from build123d import *

# Parameters (mm, degrees)
SKETCH_1_R          = 2
EXTRUDE_1_DEPTH     = 5
SKETCH_2_R          = 2.5
EXTRUDE_2_DEPTH     = 30
SKETCH_3_R          = 3.5
EXTRUDE_3_DEPTH     = 4
CUT_EXTRUDE_1_DEPTH = 3


with BuildPart() as part:
    # Эскиз1 → Бобышка-Вытянуть1 (new body)
    with BuildSketch(Plane.XY):
        Circle(SKETCH_1_R)
    extrude(amount=EXTRUDE_1_DEPTH)

    # Эскиз2 → Бобышка-Вытянуть2 (add)
    with BuildSketch(Plane.XY.offset(5)):
        Circle(SKETCH_2_R)
    extrude(amount=EXTRUDE_2_DEPTH)

    # Эскиз3 → Бобышка-Вытянуть3 (add)
    with BuildSketch(Plane.XY.offset(35)):
        Circle(SKETCH_3_R)
    extrude(amount=EXTRUDE_3_DEPTH)

    # Эскиз4 → Вырез-Вытянуть1 (cut)
    with BuildSketch(Plane.XY.offset(39)):
        Polygon((1.5, 0.866025404), (0, 1.732050808), (-1.5, 0.866025404), (-1.5, -0.866025404), (0, -1.732050808), (1.5, -0.866025404), align=None)
    extrude(amount=-CUT_EXTRUDE_1_DEPTH, mode=Mode.SUBTRACT)


solid = part.part
Check sheet for the modelled part. Datum: model origin and axes. Units: mm. A direction names the side the tool comes from. Give positions to 0.01 mm unless a question says otherwise; leave off trailing zeros. Write each loop counter-clockwise with the first axis right and the second up, starting at its lowest first coordinate (ties: lowest second). Pieces come first, ordered by that corner, then holes. Notation, with made-up numbers: (-2, 67) -> (6, 67) arc R24 cw to (6, 103) -> close; hole circle Ø10 at (-26, 10.5). An arc over 180 degrees is marked (long way). One line per item, written item: value. Start each with the question number.
Item 1: Section check C-C on z = 6. Record the cut outline in (x, y).
Item 2: Section check B-B on x = -0.5. Record the cut outline in (y, z).
Item 3: Section check A-A on y = 0. Record the cut outline in (x, z).
Item 4: Draft check along Y on faces 4 (the cylindrical face through (-0.54, -2.44, 19.79)), 5 (the flat face through (-0.74, 1.305, 37.521)), 6 (the flat face through (2, -2, 35)). Enter one of: +Y half, -Y half, draft (parallel to the pull), parting line (faces both ways), or undercut.
Item 5: Material ranges on probe 1 along X at (y, z) = (2, 31.5); probe 2 along X at (y, z) = (1.5, 10), recorded low to high. Write a range as from..to.
Item 6: Gauge pin test, flat ends, axial feed: pin 1 (0.9 mm diameter, centred on x = 0, y = 0, fed in from +Z); pin 2 (1 mm diameter, centred on y = 0.5, z = 25.5, fed in from -X). Record the tip position at first contact, or that the pin passes through.
Item 7: Section check D-D on y = 3. Record the cut outline in (x, z).
Item 8: Tool access check on faces 1 (the flat face through (-1, 2, 5)), 2 (the cylindrical face through (3.233, -1.341, 36.972)), 3 (the flat face through (0.74, -1.305, 37.521)). Record the directions out of +Z, -Z, +X, -X, +Y, -Y that give a thin tool (end or side, any length) a straight path to the whole face; none if there is none.
Results list:
1. outline: circle Ø5 at (0, 0)
2. outline: (-3.46, 35) -> (-2.45, 35) -> (-2.45, 5) -> (-1.94, 5) -> (-1.94, 0) -> (1.94, 0) -> (1.94, 5) -> (2.45, 5) -> (2.45, 35) -> (3.46, 35) -> (3.46, 39) -> (1.44, 39) -> (1.44, 36) -> (-1.44, 36) -> (-1.44, 39) -> (-3.46, 39) -> close
3. outline: (-3.5, 35) -> (-2.5, 35) -> (-2.5, 5) -> (-2, 5) -> (-2, 0) -> (2, 0) -> (2, 5) -> (2.5, 5) -> (2.5, 35) -> (3.5, 35) -> (3.5, 39) -> (1.5, 39) -> (1.5, 36) -> (-1.5, 36) -> (-1.5, 39) -> (-3.5, 39) -> close
4. face 4: parting line
4. face 5: undercut
4. face 6: draft
5. probe 1: -1.5..1.5
5. probe 2: -2..2
6. pin 1: z = 36
6. pin 2: x = -2.5
7. outline: (-1.8, 35) -> (1.8, 35) -> (1.8, 39) -> (-1.8, 39) -> close
8. face 1: -Z
8. face 2: +Z, -Z
8. face 3: +Z
